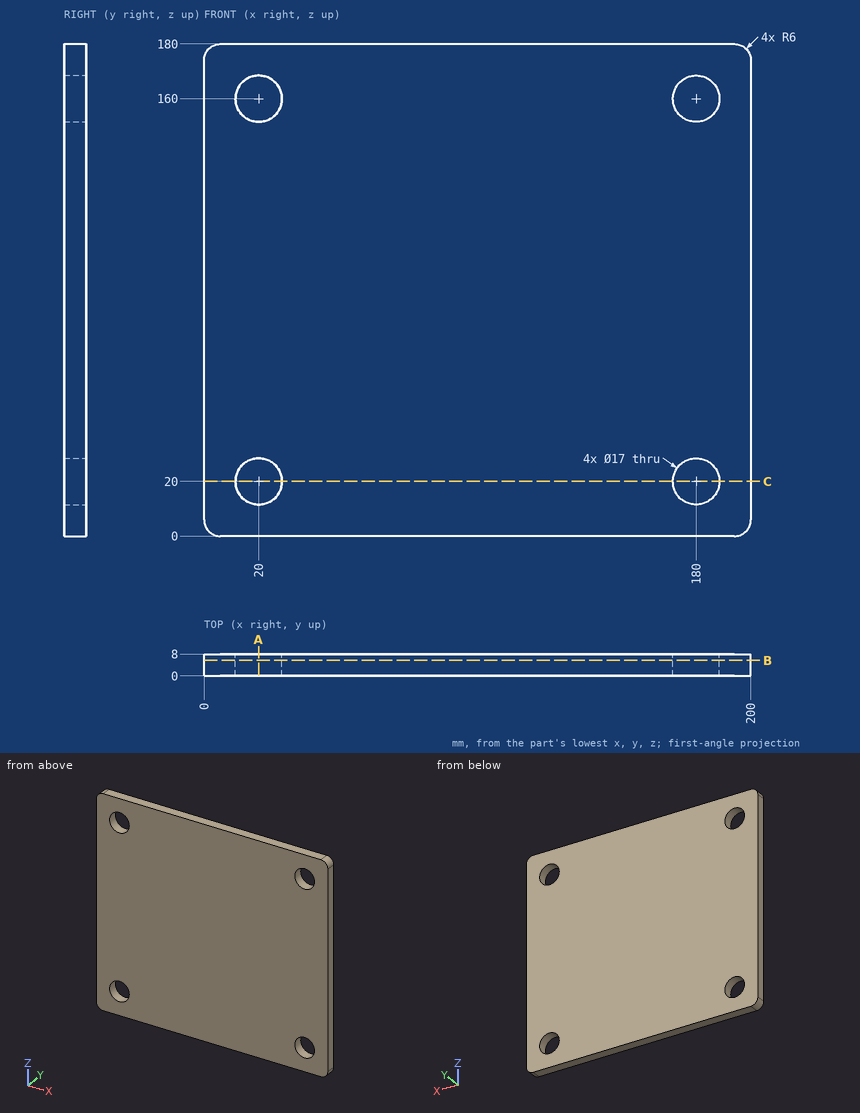
Design review of the part shown in the three views and the two pictorial views. Dimensions are in mm from the part's minimum x, y and z. Coordinates: 2 decimals unless noted, no trailing zeros. Write each loop counter-clockwise with the first axis right and the second up, starting at its lowest first coordinate (ties: lowest second). Pieces come first, ordered by that corner, then holes.
(1) For pin 1 Ø4 at (x, z) = (111, 103.5) entering from -Y, flat-tipped, find the tip position at first contact; note if it passes through.
(2) Add section B-B on y = 5.75. Give the boundary of the cut face in (x, z).
(3) Add section C-C on z = 20. Give the boundary of the cut face in (x, y), then the cut area to 3 significant figures.
(4) Add section A-A on x = 20. Give the boundary of the cut face in (y, z).
(5) Wall thickness on probe 1 along Z at (x, y) = (180, 5); probe 2 along Z at (x, y) = (14.5, 5); probe 3 along X at (y, z) = (3, 16): over which ranges is each line inside the solid? List them lowest first.
Answer sheet:
1. pin 1: stops at y = 0
2. outline: (0, 6) arc R6 ccw to (6, 0) - (194, 0) arc R6 ccw to (200, 6) - (200, 174) arc R6 ccw to (194, 180) - (6, 180) arc R6 ccw to (0, 174) - close; hole circle Ø17 at (20, 20); hole circle Ø17 at (20, 160); hole circle Ø17 at (180, 20); hole circle Ø17 at (180, 160)
3. outline: (0, 0) - (11.5, 0) - (11.5, 8) - (0, 8) - close; (28.5, 0) - (171.5, 0) - (171.5, 8) - (28.5, 8) - close; (188.5, 0) - (200, 0) - (200, 8) - (188.5, 8) - close
3. area: 1,330 mm2
4. outline: (0, 0) - (8, 0) - (8, 11.5) - (0, 11.5) - close; (0, 28.5) - (8, 28.5) - (8, 151.5) - (0, 151.5) - close; (0, 168.5) - (8, 168.5) - (8, 180) - (0, 180) - close
5. probe 1: z = 0 to 11.5, 28.5 to 151.5, 168.5 to 180
5. probe 2: z = 0 to 13.52, 26.48 to 153.52, 166.48 to 180
5. probe 3: x = 0 to 12.5, 27.5 to 172.5, 187.5 to 200
